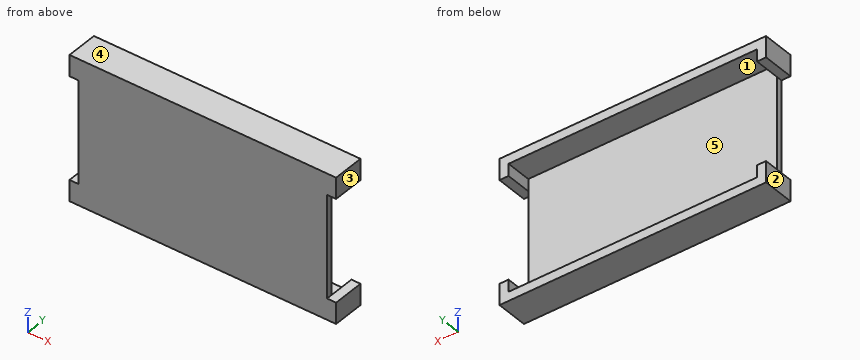
from build123d import *

# Parameters (mm, degrees)
BOSS_EXTRUDE1_DEPTH = 5.25
SKETCH1_2_W         = 41.25
SKETCH1_2_H         = 21
BOSS_EXTRUDE2_DEPTH = 1


with BuildPart() as part:
    # Sketch1 → Boss-Extrude1 (new body)
    with BuildSketch(Plane(origin=(0, 0, 0), x_dir=(1, 0, 0), z_dir=(0, 1, 0))):
        Polygon((20.625, -10.5), (0, -10.5), (0, -12), (22.125, -12), (22.125, -8.5), (20.625, -8.5), align=None)
        Polygon((-20.625, -8.5), (-22.125, -8.5), (-22.125, -12), (0, -12), (0, -10.5), (-20.625, -10.5), align=None)
        Polygon((0, 12), (-22.125, 12), (-22.125, 8.5), (-20.625, 8.5), (-20.625, 10.5), (0, 10.5), align=None)
        Polygon((22.125, 12), (0, 12), (0, 10.5), (20.625, 10.5), (20.625, 8.5), (22.125, 8.5), align=None)
    extrude(amount=BOSS_EXTRUDE1_DEPTH)

    # Sketch1_2 → Boss-Extrude2 (add)
    with BuildSketch(Plane(origin=(0, 0, 0), x_dir=(1, 0, 0), z_dir=(0, 1, 0))):
        Rectangle(SKETCH1_2_W, SKETCH1_2_H)
    extrude(amount=BOSS_EXTRUDE2_DEPTH)


solid = part.part
The listing builds one solid part. Answer for the finished solid, in the listing's coordinates (mm). Face numbers are marked on the shaded views. A direction names the side the tool comes from. Coordinates: 2 decimals unless noted, no trailing zeros. Write each loop counter-clockwise with the first axis right and the second up, starting at its lowest first coordinate (ties: lowest second). Pieces come first, ordered by that corner, then holes. Notation, with made-up numbers: M 82.5,-13 L 140.5,-13 A25 ccw 140.5,16 Z; hole C 16.25,39.25 d1. An arc over 180 degrees is marked long. Use one line per item in the form item = value.
Item 1: Find section A-A, the plane y = 2.6. Give the vertices of the cut face in (x, z) (3 decimals).
Model answer:
outline = M -22.125,-12 L 22.125,-12 L 22.125,-8.5 L 20.625,-8.5 L 20.625,-10.5 L -20.625,-10.5 L -20.625,-8.5 L -22.125,-8.5 Z; M -22.125,8.5 L -20.625,8.5 L -20.625,10.5 L 20.625,10.5 L 20.625,8.5 L 22.125,8.5 L 22.125,12 L -22.125,12 Z
Item 2: Find the intervals of material crossed by probe 1 along X at (y, z) = (1.8, 10) (3 decimals); probe 2 along Z at (x, y) = (6.5, 2.8); probe 3 along Y at (x, z) = (-10, 4.25), in increasing order.
Model answer:
probe_1 = -22.125 to -20.625, 20.625 to 22.125
probe_2 = -12 to -10.5, 10.5 to 12
probe_3 = 0 to 1
Item 3: Find section B-B, the plane z = 9.25. Give the vertices of the cut face in (x, y) (3 decimals), plus the area to 3 significant figures.
Model answer:
outline = M -22.125,0 L 22.125,0 L 22.125,5.25 L 20.625,5.25 L 20.625,1 L -20.625,1 L -20.625,5.25 L -22.125,5.25 Z
area = 57.0 mm2
Item 4: Find section D-D, the plane z = 3.5. Give the vertices of the cut face in (x, y) (3 decimals).
Model answer:
outline = M -20.625,0 L 20.625,0 L 20.625,1 L -20.625,1 Z
Item 5: Find section C-C, the plane x = -10. Give the vertices of the cut face in (y, z), plus the area to 4 significant figures.
Model answer:
outline = M 0,-12 L 5.25,-12 L 5.25,-10.5 L 1,-10.5 L 1,10.5 L 5.25,10.5 L 5.25,12 L 0,12 Z
area = 36.75 mm2
Item 6: Given P1, Ø2, axis at x = -0.5, z = -2, coming from the +Y side; P2, Ø1.1, axis at y = 0.5, z = 0.5, coming from the +X side (3 decimals), each flat-ended and moving along its own axis, determine where each tip first touches the part or whether it passes through.
Model answer:
P1 = 1
P2 = 20.625
Item 7: For the marked faces 1 and 2, determine the directions among +Z, -Z, +X, -X, +Y, -Y from which every point of the face is accessible in a straight line to the end or side of a thin tool.
Model answer:
face_1 = +Y
face_2 = +Z, -Z, -X, +Y, -Y
Item 8: The mould has two halves that part along X. Classify the marked faces 3, 4 and 5: released by +X, released by -X, zero draft, split by the parting line, or undercut.
Model answer:
face_3 = released by +X
face_4 = zero draft
face_5 = undercut
